CAD build for the part. Positions are in the model's coordinates, mm. A direction names the side the tool comes from. Coordinates: 2 decimals unless noted, no trailing zeros. Loops run counter-clockwise (first coordinate to the right, second up) from the corner with the lowest first, then second, coordinate; pieces in that order, holes last. Notation, with made-up numbers: (10, 14) -> (48, 14) arc R33 cw to (48, 46) -> close; hole circle Ø1 at (46.5, -20.75). An arc over 180 degrees is marked (long way). Write each question's results on one line, items separated by ' | '.
from build123d import *

# Parameters (mm, degrees)
SKETCH1_W                     = 100
SKETCH1_H                     = 107
BOSS_EXTRUDE1_DEPTH           = 3
CUT_EXTRUDE_THIN2_START       = -3
CUT_EXTRUDE_THIN2_OUTLINE_W   = 5.933508572
CUT_EXTRUDE_THIN2_OUTLINE_H   = 7
CUT_EXTRUDE_THIN2_OUTLINE_W_2 = 74.23028827
CUT_EXTRUDE_THIN2_OUTLINE_W_3 = 9.836203158
CUT_EXTRUDE_THIN2_DEPTH       = 3


# Read off the part's stored shape, not the designer's step: Cut-Extrude-Thin2
with BuildPart() as part:
    # Sketch1 → Boss-Extrude1 (new body)
    with BuildSketch(Plane.XY):
        with Locations((50, -53.5)):
            Rectangle(SKETCH1_W, SKETCH1_H)
    extrude(amount=BOSS_EXTRUDE1_DEPTH)

    # Cut-Extrude-Thin2 outline → Cut-Extrude-Thin2 (cut)
    with BuildSketch(Plane.XY.offset(3).offset(CUT_EXTRUDE_THIN2_START)):
        with Locations((2.966754286, -103.5)):
            Rectangle(CUT_EXTRUDE_THIN2_OUTLINE_W, CUT_EXTRUDE_THIN2_OUTLINE_H)
        with Locations((48.048652707, -103.5)):
            Rectangle(CUT_EXTRUDE_THIN2_OUTLINE_W_2, CUT_EXTRUDE_THIN2_OUTLINE_H)
        with Locations((2.966754286, -3.5)):
            Rectangle(CUT_EXTRUDE_THIN2_OUTLINE_W, CUT_EXTRUDE_THIN2_OUTLINE_H)
        with Locations((95.081898421, -103.5)):
            Rectangle(CUT_EXTRUDE_THIN2_OUTLINE_W_3, CUT_EXTRUDE_THIN2_OUTLINE_H)
        with Locations((48.048652707, -3.5)):
            Rectangle(CUT_EXTRUDE_THIN2_OUTLINE_W_2, CUT_EXTRUDE_THIN2_OUTLINE_H)
        with Locations((95.081898421, -3.5)):
            Rectangle(CUT_EXTRUDE_THIN2_OUTLINE_W_3, CUT_EXTRUDE_THIN2_OUTLINE_H)
    extrude(amount=CUT_EXTRUDE_THIN2_DEPTH, mode=Mode.SUBTRACT)


solid = part.part
1) Two-plate mould, pull along X, no slides. Class faces 5 (the flat face through (85.164, -4, 1)), 6 (the flat face through (95, -7, 1)), 7 (the flat face through (5.934, -104, 1)): pulls with the +X half, pulls with the -X half, needs draft (parallel to the pull), parting line crosses it, or undercut.
Outcome:
face 5: undercut | face 6: needs draft | face 7: pulls with the -X half
2) Drill centre lines: L1, parallel to X at y = -6, z = 1.9; L2, parallel to Y at x = 36, z = 0.5. Where is each one in solid material? Low to high. Write a range as from..to.
Outcome:
L1: x = 5.93..10.93, 85.16..90.16 | L2: y = -100..-7
3) Slice it at A-A (z = 1.2). Write the cut outline in (x, y).
Outcome:
outline: (0, -100) -> (5.93, -100) -> (5.93, -107) -> (10.93, -107) -> (10.93, -100) -> (85.16, -100) -> (85.16, -107) -> (90.16, -107) -> (90.16, -100) -> (100, -100) -> (100, -7) -> (90.16, -7) -> (90.16, 0) -> (85.16, 0) -> (85.16, -7) -> (10.93, -7) -> (10.93, 0) -> (5.93, 0) -> (5.93, -7) -> (0, -7) -> close
4) Pin check, flat tips, straight feed: pin 1 (1.5 mm diameter, centred on x = 4, z = 2, fed in from +Y); pin 2 (0.9 mm diameter, centred on y = -4, z = 2, fed in from +X); pin 3 (0.9 mm diameter, centred on y = -103, z = 1, fed in from -X). Stop position of each tip, or through.
Outcome:
pin 1: stops at y = -7 | pin 2: stops at x = 90.16 | pin 3: stops at x = 5.93
5) Slice it at B-B (x = 16.5). Write the cut outline in (y, z).
Outcome:
outline: (-100, 0) -> (-7, 0) -> (-7, 3) -> (-100, 3) -> close
6) Which spindle directions (+Z, -Z, +X, -X, +Y, -Y) get a long thin tool onto all of the face, cutting with end or side? Do faces 1 (the flat face through (10.934, -4, 1)), 2 (the flat face through (48, -100, 1)), 3 (the flat face through (90.164, -4, 1)), 4 (the flat face through (3, -100, 1)). Say none if no direction does.
Outcome:
face 1: +Z, -Z, +Y | face 2: +Z, -Z, -Y | face 3: +Z, -Z, +X, +Y | face 4: +Z, -Z, -X, -Y
